```python
from build123d import *

# Parameters (mm, degrees)
SKETCH1_R           = 12.5
SKETCH1_R_2         = 2.5
SKETCH1_RX          = 2
SKETCH1_RY          = 1
BOSS_EXTRUDE1_DEPTH = 2


with BuildPart() as part:
    # Sketch1 → Boss-Extrude1 (new body)
    with BuildSketch(Plane.XY):
        Circle(SKETCH1_R)
        Circle(SKETCH1_R_2, mode=Mode.SUBTRACT)
        with Locations(Location((0, 9.375), (0, 0, -90))):
            Ellipse(SKETCH1_RX, SKETCH1_RY, mode=Mode.SUBTRACT)
        with Locations(Location((2.897034322, 8.91615484), (0, 0, 72))):
            Ellipse(SKETCH1_RX, SKETCH1_RY, mode=Mode.SUBTRACT)
        with Locations(Location((5.51048674, 7.584534322), (0, 0, 54))):
            Ellipse(SKETCH1_RX, SKETCH1_RY, mode=Mode.SUBTRACT)
        with Locations(Location((7.584534322, 5.51048674), (0, 0, -144))):
            Ellipse(SKETCH1_RX, SKETCH1_RY, mode=Mode.SUBTRACT)
        with Locations(Location((8.91615484, 2.897034322), (0, 0, 18))):
            Ellipse(SKETCH1_RX, SKETCH1_RY, mode=Mode.SUBTRACT)
        with Locations(Location((9.375, 0), (0, 0, 180))):
            Ellipse(SKETCH1_RX, SKETCH1_RY, mode=Mode.SUBTRACT)
        with Locations(Location((8.91615484, -2.897034322), (0, 0, -18))):
            Ellipse(SKETCH1_RX, SKETCH1_RY, mode=Mode.SUBTRACT)
        with Locations(Location((7.584534322, -5.51048674), (0, 0, -36))):
            Ellipse(SKETCH1_RX, SKETCH1_RY, mode=Mode.SUBTRACT)
        with Locations(Location((5.51048674, -7.584534322), (0, 0, 126))):
            Ellipse(SKETCH1_RX, SKETCH1_RY, mode=Mode.SUBTRACT)
        with Locations(Location((2.897034322, -8.91615484), (0, 0, 108))):
            Ellipse(SKETCH1_RX, SKETCH1_RY, mode=Mode.SUBTRACT)
        with Locations(Location((0, -9.375), (0, 0, 90))):
            Ellipse(SKETCH1_RX, SKETCH1_RY, mode=Mode.SUBTRACT)
        with Locations(Location((-2.897034322, -8.91615484), (0, 0, 72))):
            Ellipse(SKETCH1_RX, SKETCH1_RY, mode=Mode.SUBTRACT)
        with Locations(Location((-5.51048674, -7.584534322), (0, 0, 54))):
            Ellipse(SKETCH1_RX, SKETCH1_RY, mode=Mode.SUBTRACT)
        with Locations(Location((-7.584534322, -5.51048674), (0, 0, -144))):
            Ellipse(SKETCH1_RX, SKETCH1_RY, mode=Mode.SUBTRACT)
        with Locations(Location((-8.91615484, -2.897034322), (0, 0, 18))):
            Ellipse(SKETCH1_RX, SKETCH1_RY, mode=Mode.SUBTRACT)
        with Locations(Location((-9.375, 0), (0, 0, 0))):
            Ellipse(SKETCH1_RX, SKETCH1_RY, mode=Mode.SUBTRACT)
        with Locations(Location((-8.91615484, 2.897034322), (0, 0, 162))):
            Ellipse(SKETCH1_RX, SKETCH1_RY, mode=Mode.SUBTRACT)
        with Locations(Location((-7.584534322, 5.51048674), (0, 0, -36))):
            Ellipse(SKETCH1_RX, SKETCH1_RY, mode=Mode.SUBTRACT)
        with Locations(Location((-5.51048674, 7.584534322), (0, 0, -54))):
            Ellipse(SKETCH1_RX, SKETCH1_RY, mode=Mode.SUBTRACT)
        with Locations(Location((-2.897034322, 8.91615484), (0, 0, -72))):
            Ellipse(SKETCH1_RX, SKETCH1_RY, mode=Mode.SUBTRACT)
    extrude(amount=BOSS_EXTRUDE1_DEPTH)


solid = part.part
```
Design review of the part built by this model. Coordinates are the model's own, in mm. Give positions to 0.01 mm unless a question says otherwise; leave off trailing zeros. Return JSON: item names as keys, results as strings. Group by question number.
(1) Mouldability with a two-part tool opening along X and no side actions: class faces 1 (the cylindrical face through (11.923, 3.755, 0.986)), 2 (the flat face through (0, -3, 2)), 3 (the cylindrical face through (-0.54, -2.44, 0.99)) as +X half, -X half, draft (parallel to the pull), parting line (faces both ways), or undercut.
(2) Insertion check: pin 1 (1 mm diameter, centred on y = 7.5, z = 1, fed in from +X); pin 2 (1 mm diameter, centred on y = 5.5, z = 1.5, fed in from -X). Each pin has a flat end and moves straight along its axis. Give the tip position at first contact, or say it passes through.
(3) To check wall thickness, follow probe 1 along X at (y, z) = (-7.75, 0.45); probe 2 along Y at (x, z) = (10, 1.2); probe 3 along X at (y, z) = (-4.75, 0.45). State the ranges of each line that lie inside material, in increasing order.
(4) We need section A-A, the plane x = 0. Give the number of separate pieces and of enclosed holes in the cut face, then the cut area to 3 significant figures.
Reported:
{
 "1": {"face 1": "parting line", "face 2": "draft", "face 3": "undercut"},
 "2": {"pin 1": "stops at x = 10.36", "pin 2": "stops at x = -11.46"},
 "3": {"probe 1": "x = -9.81 to -6.75, -4.43 to -3.45, -1.79 to -0.58, 0.58 to 1.79, 3.45 to 4.43, 6.75 to 9.81", "probe 2": "y = -7.5 to -4.01, -2.3 to -0.95, 0.95 to 2.3, 4.01 to 7.5", "probe 3": "x = -11.56 to -8.24, -5.87 to 5.87, 8.24 to 11.56"},
 "4": {"separate pieces": "4", "enclosed holes": "0", "area": "24.0 mm2"}
}
